Design review of the part shown in the three views and the two pictorial views. Dimensions are in mm from the part's minimum x, y and z. Round coordinates to 2 decimals unless told otherwise and drop trailing zeros. Write each loop counter-clockwise with the first axis right and the second up, starting at its lowest first coordinate (ties: lowest second). Pieces come first, ordered by that corner, then holes. Notation, with made-up numbers: (44.25, 58.5) - (98.25, 58.5) arc R26 cw to (98.25, 96.5) - close; hole circle Ø7 at (-17, 78.5). An arc over 180 degrees is marked (long way). Use one line per item in the form item = value.
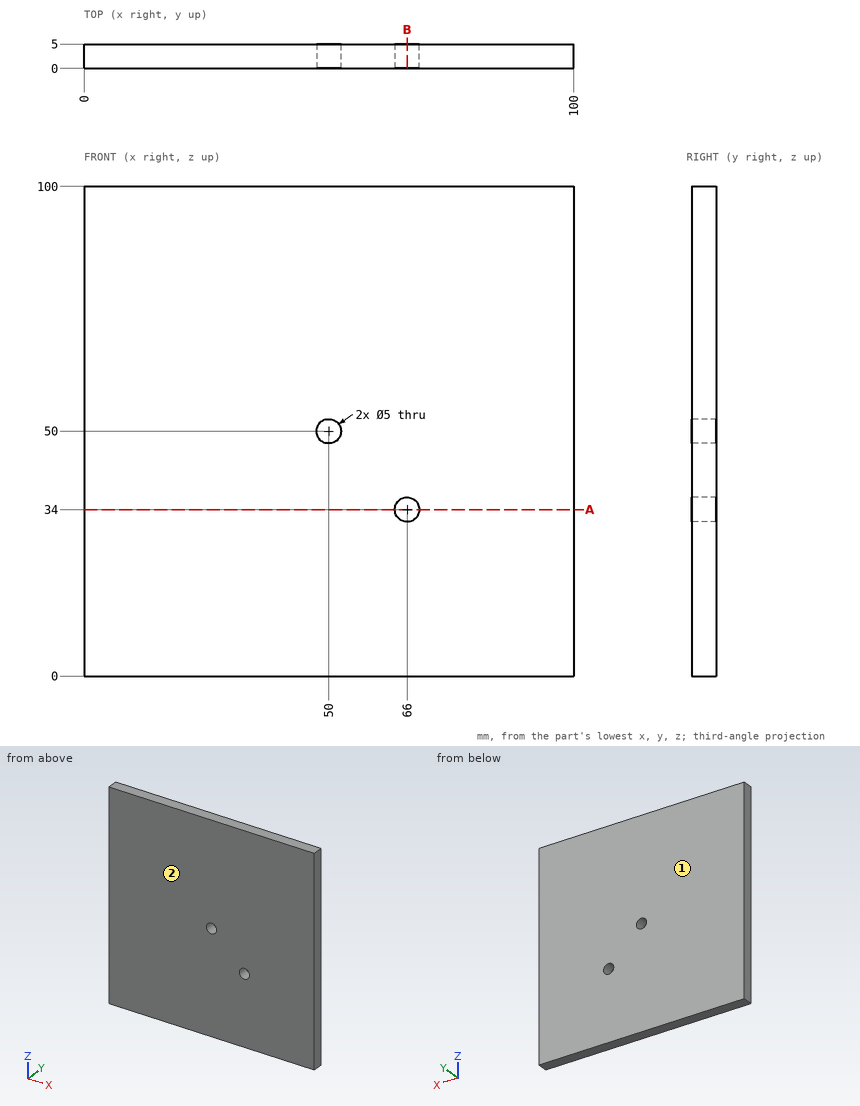
Q1. For P1, Ø3, axis at x = 66, z = 34, coming from the -Y side; P2, Ø3, axis at y = 2, z = 90, coming from the -X side, all flat-tipped, find the tip position at first contact; note any pin that passes through.
Calculated:
P1 = through
P2 = 0
Q2. We need section B-B on x = 66. Write out the cut boundary in (y, z).
Calculated:
outline = (0, 0) - (5, 0) - (5, 31.5) - (0, 31.5) - close; (0, 36.5) - (5, 36.5) - (5, 100) - (0, 100) - close
Q3. To check wall thickness, follow line 1 along Z through (x, y) = (66, 2.25); line 2 along X through (y, z) = (2.55, 34); line 3 along Z through (x, y) = (50, 3.6). State the ranges of each line that lie inside material, in increasing order. Write a range as from..to.
Calculated:
line_1 = 0..31.5, 36.5..100
line_2 = 0..63.5, 68.5..100
line_3 = 0..47.5, 52.5..100
Q4. Draft analysis for pull direction Y (two halves, no side actions). For the marked faces 1 and 2, state which applies: released by +Y, released by -Y, zero draft, split by the parting line, or undercut.
Calculated:
face_1 = released by +Y
face_2 = released by -Y
Q5. We need section A-A on z = 34. Write out the cut boundary in (x, y), then the cut area to 3 significant figures.
Calculated:
outline = (0, 0) - (63.5, 0) - (63.5, 5) - (0, 5) - close; (68.5, 0) - (100, 0) - (100, 5) - (68.5, 5) - close
area = 475 mm2
